```python
from build123d import *

# Parameters (mm, degrees)
PAD006_DEPTH    = 10
POCKET_DEPTH    = 3
POCKET001_DEPTH = 8.75
POCKET002_DEPTH = 10.001
SKETCH071_R     = 1.25
POCKET032_DEPTH = 5


with BuildPart() as part:
    # Sketch006 → Pad006 (new body)
    with BuildSketch(Plane.XY):
        with BuildLine():
            Line((1, 0), (374, 0))
            ThreePointArc((374, 0), (374.707107, 0.292893), (375, 1))
            Line((375, 1), (375, 228.5))
            ThreePointArc((375, 228.5), (374.707107, 229.207107), (374, 229.5))
            Line((374, 229.5), (1, 229.5))
            ThreePointArc((1, 229.5), (0.292893, 229.207107), (0, 228.5))
            Line((0, 228.5), (0, 1))
            ThreePointArc((0, 1), (0.292893, 0.292893), (1, 0))
        make_face()
    extrude(amount=-PAD006_DEPTH)

    # Sketch007 → Pocket (cut)
    with BuildSketch(Plane.XY):
        with BuildLine():
            Line((4, 3), (371, 3))
            ThreePointArc((371, 3), (371.707107, 3.292893), (372, 4))
            Line((372, 4), (372, 225.5))
            ThreePointArc((372, 225.5), (371.707107, 226.207107), (371, 226.5))
            Line((371, 226.5), (4, 226.5))
            ThreePointArc((4, 226.5), (3.292893, 226.207107), (3, 225.5))
            Line((3, 225.5), (3, 4))
            ThreePointArc((3, 4), (3.292893, 3.292893), (4, 3))
        make_face()
    extrude(amount=-POCKET_DEPTH, mode=Mode.SUBTRACT)

    # Sketch008 → Pocket001 (cut)
    with BuildSketch(Plane.XY):
        with BuildLine():
            Line((10.05, 222.45), (368.95, 222.45))
            ThreePointArc((369.45, 221.95), (369.303553, 222.303553), (368.95, 222.45))
            Line((369.45, 221.95), (369.45, 15.55))
            ThreePointArc((368.95, 15.05), (369.303553, 15.196447), (369.45, 15.55))
            Line((368.95, 15.05), (339.95, 15.05))
            ThreePointArc((339.95, 15.05), (339.596447, 14.903553), (339.45, 14.55))
            Line((339.45, 14.55), (339.45, 4.85))
            ThreePointArc((338.95, 4.35), (339.303553, 4.496447), (339.45, 4.85))
            Line((338.95, 4.35), (40.05, 4.35))
            ThreePointArc((39.55, 4.85), (39.696447, 4.496447), (40.05, 4.35))
            Line((39.55, 4.85), (39.55, 14.05))
            ThreePointArc((39.55, 14.05), (39.403553, 14.403553), (39.05, 14.55))
            Line((39.05, 14.55), (10.05, 14.55))
            ThreePointArc((9.55, 15.05), (9.696447, 14.696447), (10.05, 14.55))
            Line((9.55, 15.05), (9.55, 221.95))
            ThreePointArc((10.05, 222.45), (9.696447, 222.303553), (9.55, 221.95))
        make_face()
    extrude(amount=-POCKET001_DEPTH, mode=Mode.SUBTRACT)

    # Sketch009 → Pocket002 (cut, through all)
    with BuildSketch(Plane.XY):
        with BuildLine():
            Line((19.55, 45.05), (267.55, 45.05))
            ThreePointArc((267.55, 45.05), (268.257107, 45.342893), (268.55, 46.05))
            Line((268.55, 46.05), (268.55, 99.05))
            ThreePointArc((268.55, 99.05), (268.257107, 99.757107), (267.55, 100.05))
            Line((267.55, 100.05), (19.55, 100.05))
            ThreePointArc((19.55, 100.05), (18.842893, 99.757107), (18.55, 99.05))
            Line((18.55, 99.05), (18.55, 46.05))
            ThreePointArc((18.55, 46.05), (18.842893, 45.342893), (19.55, 45.05))
        make_face()
    extrude(amount=-POCKET002_DEPTH, mode=Mode.SUBTRACT)

    # Sketch071 (on DatumPlane) → Pocket032 (cut)
    with BuildSketch(Plane.XY.offset(-10)):
        with Locations((5, 221.5)):
            Circle(SKETCH071_R)
        with Locations((5, 8)):
            Circle(SKETCH071_R)
        with Locations((370, 8)):
            Circle(SKETCH071_R)
        with Locations((370, 221.5)):
            Circle(SKETCH071_R)
        with Locations((370, 114.75)):
            Circle(SKETCH071_R)
        with Locations((162.5, 196)):
            Circle(SKETCH071_R)
        with Locations((212.5, 196)):
            Circle(SKETCH071_R)
        with Locations((90, 196)):
            Circle(SKETCH071_R)
        with Locations((285, 196)):
            Circle(SKETCH071_R)
        with Locations((187.5, 5)):
            Circle(SKETCH071_R)
    extrude(amount=POCKET032_DEPTH, mode=Mode.SUBTRACT)


solid = part.part
```
Here's how the part is built. I have some questions about the finished solid (model axes, mm). A direction names the side the tool comes from. Coordinates: 2 decimals unless noted, no trailing zeros. Order: outer loops, then holes, each group sorted by start corner. A loop starts at its lowest first (then second) coordinate and runs counter-clockwise, first axis right, second up.
Item 1: If we section it at C-C, the plane x = 326.5: List the corners of the cut face in (y, z) for me, then the cut area to 3 significant figures.
Response values:
outline: (0, -10) - (229.5, -10) - (229.5, 0) - (226.5, 0) - (226.5, -3) - (222.45, -3) - (222.45, -8.75) - (4.35, -8.75) - (4.35, -3) - (3, -3) - (3, 0) - (0, 0) - close
area: 370 mm2
Item 2: If we section it at D-D, the plane y = 27.5: List the corners of the cut face in (x, z) for me.
Response values:
outline: (0, -10) - (375, -10) - (375, 0) - (372, 0) - (372, -3) - (369.45, -3) - (369.45, -8.75) - (9.55, -8.75) - (9.55, -3) - (3, -3) - (3, 0) - (0, 0) - close
Item 3: If we section it at A-A, the plane y = 84.5: List the corners of the cut face in (x, z) for me.
Response values:
outline: (0, -10) - (18.55, -10) - (18.55, -8.75) - (9.55, -8.75) - (9.55, -3) - (3, -3) - (3, 0) - (0, 0) - close; (268.55, -10) - (375, -10) - (375, 0) - (372, 0) - (372, -3) - (369.45, -3) - (369.45, -8.75) - (268.55, -8.75) - close
Item 4: I'm going to push flat-ended pins straight in: pin 1 Ø2 at (x, y) = (370.5, 114.5) entering from -Z; pin 2 Ø0.8 at (x, y) = (5, 7.5) entering from -Z; pin 3 Ø3 at (x, y) = (5, 221.5) entering from +Z. Where does each tip first touch, or does it pass through?
Response values:
pin 1: stops at z = -10
pin 2: stops at z = -5
pin 3: stops at z = -3
Item 5: If we section it at B-B, the plane z = -1.5: List the corners of the cut face in (x, y) for me.
Response values:
outline: (0, 1) arc R1 ccw to (1, 0) - (374, 0) arc R1 ccw to (375, 1) - (375, 228.5) arc R1 ccw to (374, 229.5) - (1, 229.5) arc R1 ccw to (0, 228.5) - close; hole (3, 4) arc R1 ccw to (4, 3) - (371, 3) arc R1 ccw to (372, 4) - (372, 225.5) arc R1 ccw to (371, 226.5) - (4, 226.5) arc R1 ccw to (3, 225.5) - close
Item 6: Thinking about a two-plate mould opening in Y: for faces 3 (the face through (185, 0, -5)), 4 (the face through (190, 229.5, -5)), 5 (the face through (375, 113, -5)), 6 (the face through (105, 223, -3)), which applies, pulls with the +Y half, pulls with the -Y half, needs draft (parallel to the pull), parting line crosses it, or undercut?
Response values:
face 3: pulls with the -Y half
face 4: pulls with the +Y half
face 5: needs draft
face 6: undercut
Item 7: Which directions (+Z, -Z, +X, -X, +Y, -Y) give clear straight access to the entire face, cutting with the end or side of a thin tool? Please do faces 1 (the face through (185, 116, -10)), 2 (the face through (192, 115, -8.75)).
Response values:
face 1: -Z, +X, -X, +Y, -Y
face 2: +Z
Item 8: I need wall thicknesses on probe 1 along Y at (x, z) = (90, -9.45); probe 2 along X at (y, z) = (196, -9.1); probe 3 along X at (y, z) = (76, -9.5). Which ranges of each line are inside material? Lowest first, please.
Response values:
probe 1: y = 0 to 45.05, 100.05 to 194.75, 197.25 to 229.5
probe 2: x = 0 to 88.75, 91.25 to 161.25, 163.75 to 211.25, 213.75 to 283.75, 286.25 to 375
probe 3: x = 0 to 18.55, 268.55 to 375
